Can you work these out from the model? Positions are in its coordinate system, mm. Coordinates: 2 decimals unless noted, no trailing zeros. Order: outer loops, then holes, each group sorted by start corner. A loop starts at its lowest first (then second) coordinate and runs counter-clockwise, first axis right, second up. Notation, with made-up numbers: M 27,-15.5 L 66,-15.5 A31 ccw 66,20.5 Z; hole C -4.5,61.5 d8. An arc over 180 degrees is marked long. Answer as a JSON object with one key per item and string values.
Autodesk Inventor part; units mm, degrees
ref_plane "YZ Plane" through (0, 0, 0) normal (1, 0, 0) x (0, 1, 0)
ref_plane "XZ Plane" through (0, 0, 0) normal (0, 1, 0) x (-1, 0, 0)
ref_plane "XY Plane" through (0, 0, 0) normal (0, 0, 1) x (1, 0, 0)
sketch "Sketch1" plane through (0, 0, 0) normal (0, 0, 1) x (1, 0, 0)
  line L0 (-25, -9.5) -> (25, -9.5)
  line L1 (25, -9.5) -> (25, 9.5)
  line L2 (25, 9.5) -> (-25, 9.5)
  line L3 (-25, 9.5) -> (-25, -9.5)
  line L4 (-25, -9.5) -> (25, 9.5) construction
  line L5 (25, -9.5) -> (-25, 9.5) construction
  point P0 (0, 0)
  dimension "d0" = 50
  dimension "d1" = 19
extrude "Extrusion1" add sketch "Sketch1" along normal blind 6
sketch "Sketch2" plane through (0, 0, 6) normal (0, 0, 1) x (1, 0, 0)
  line L0 (-25, -9.5) -> (25, -9.5)
  line L1 (-25, 9.5) -> (-25, -9.5)
  line L2 (25, -9.5) -> (25, 9.5)
  point P0 (0, 0)
  point P1 (-18, -4.5)
  point P2 (18, -4.5)
  dimension "d4" = 5
  dimension "d5" = 5
  dimension "d6" = 7
  dimension "d7" = 7
hole "Hole1" at (-18, -4.5, 6) at (18, -4.5, 6) direction (0, 0, -1) diameter 4.134 depth 6
properties part number "Funrungesch" material "Steel, Mild"
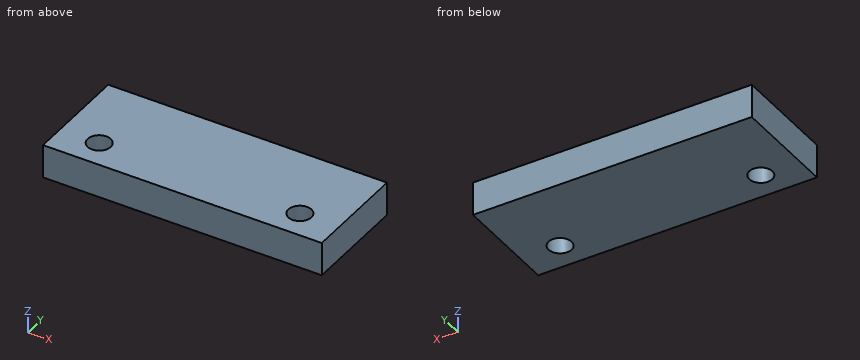
Item 1: I want a section at C-C, the plane y = -3.5. Write out the boundary of the cut face in (x, z).
Answers follow:
{"outline": "M -25,0 L -19.81,0 L -19.81,6 L -25,6 Z; M -16.19,0 L 16.19,0 L 16.19,6 L -16.19,6 Z; M 19.81,0 L 25,0 L 25,6 L 19.81,6 Z"}
Item 2: Please list where these lines run through material, in increasing order: line 1 (X direction, y = -4.5, z = 4.15); line 2 (Y direction, x = -18, z = 1.7); line 3 (X direction, y = -3.75, z = 4.65).
Answers follow:
{"line 1": "x = -25 to -20.07, -15.93 to 15.93, 20.07 to 25", "line 2": "y = -9.5 to -6.57, -2.43 to 9.5", "line 3": "x = -25 to -19.93, -16.07 to 16.07, 19.93 to 25"}
Item 3: I want a section at B-B, the plane x = 18. Write out the boundary of the cut face in (y, z).
Answers follow:
{"outline": "M -9.5,0 L -6.57,0 L -6.57,6 L -9.5,6 Z; M -2.43,0 L 9.5,0 L 9.5,6 L -2.43,6 Z"}
Item 4: I want a section at A-A, the plane z = 2.4. Write out the boundary of the cut face in (x, y).
Answers follow:
{"outline": "M -25,-9.5 L 25,-9.5 L 25,9.5 L -25,9.5 Z; hole C -18,-4.5 d4.13; hole C 18,-4.5 d4.13"}
